For this review, take the finished solid that the model builds, in its own axes (mm). A direction names the side the tool comes from. Round coordinates to 2 decimals unless told otherwise and drop trailing zeros. Write item = value, one per line. Start each with the question number.
```python
from build123d import *

# Parameters (mm, degrees)
SKETCH004_W     = 168
SKETCH004_H     = 180
PAD002_DEPTH    = 45
SKETCH005_R     = 3
POCKET002_DEPTH = 8
FILLET001_R     = 5


with BuildPart() as part:
    # Sketch004 → Pad002 (new body)
    with BuildSketch(Plane.XY):
        Rectangle(SKETCH004_W, SKETCH004_H)
    extrude(amount=PAD002_DEPTH)

    # Sketch005 (on Face2 of Pad002) → Pocket002 (cut)
    with BuildSketch(Plane.YZ.offset(84)):
        with Locations((15, 18)):
            Circle(SKETCH005_R)
    pocket002 = extrude(amount=-POCKET002_DEPTH, mode=Mode.SUBTRACT)

    # Mirrored: Pocket002 across YZ
    add(pocket002.mirror(Plane.YZ), mode=Mode.SUBTRACT)

    # Fillet001
    fillet001_edges = [part.edges().sort_by_distance(p)[0] for p in [
        (84, -90, 22.5),
        (-84, -90, 22.5),
        (0, -90, 0),
        (0, -90, 45),
    ]]
    fillet(fillet001_edges, radius=FILLET001_R)


solid = part.part
```
(1) Wall thickness on L1, parallel to Z at x = 79.75, y = 15; L2, parallel to Y at x = 47.5, z = 43: over which ranges is each line inside the solid? List them lowest first.
(2) For pin 1 Ø5.5 at (y, z) = (15, 18) entering from -X, flat-tipped, find the tip position at first contact; note if it passes through.
(3) Draft analysis for pull direction Y (two halves, no side actions). For faces 4 (the cylindrical face through (-80.1, 12.6, 16.2)), 5 (the cylindrical face through (1, -89, 2)), 6 (the flat face through (84, 1, 22)), state which applies: +Y half, -Y half, draft (parallel to the pull), parting line (faces both ways), or undercut.
(4) Tool access review of faces 1 (the cylindrical face through (-83, -88, 23)), 2 (the cylindrical face through (80.1, 12.6, 16.2)), 3 (the flat face through (-76, 15, 18)): name each direction out of +Z, -Z, +X, -X, +Y, -Y from which nothing blocks a thin tool from reaching the whole face with its end or side.
Answer sheet:
q1.L1 = 0 to 15, 21 to 45
q1.L2 = -89 to 90
q2.pin_1 = -76
q3.face_4 = undercut
q3.face_5 = -Y half
q3.face_6 = draft
q4.face_1 = +Z, -Z, -X, -Y
q4.face_2 = +X
q4.face_3 = -X
